Part model, mm, in its own coordinate system. A direction names the side the tool comes from. Round coordinates to 2 decimals unless told otherwise and drop trailing zeros. Order: outer loops, then holes, each group sorted by start corner. A loop starts at its lowest first (then second) coordinate and runs counter-clockwise, first axis right, second up. Notation, with made-up numbers: (-30.5, -12) -> (-17.5, -12) arc R9 ccw to (-17.5, 3) -> close; hole circle Ø9 at (-10.5, 71). An arc over 180 degrees is marked (long way). Answer as a JSON object with one key per item and string values. Group by question number.
```python
from build123d import *

# Parameters (mm, degrees)
SKETCH1_W           = 90
SKETCH1_H           = 140
BOSS_EXTRUDE1_DEPTH = 5
SKETCH2_W           = 80
SKETCH2_H           = 85
CUT_EXTRUDE1_DEPTH  = 2
SKETCH3_W           = 90
SKETCH3_H           = 3
BOSS_EXTRUDE2_DEPTH = 50
SKETCH4_W           = 2
SKETCH4_H           = 134
BOSS_EXTRUDE3_DEPTH = 50
SKETCH5_R           = 4
CUT_EXTRUDE2_DEPTH  = 3
SKETCH6_R           = 4
CUT_EXTRUDE3_DEPTH  = 3


with BuildPart() as part:
    # Sketch1 → Boss-Extrude1 (new body)
    with BuildSketch(Plane(origin=(0, 0, 0), x_dir=(1, 0, 0), z_dir=(0, 1, 0))):
        Rectangle(SKETCH1_W, SKETCH1_H)
    extrude(amount=BOSS_EXTRUDE1_DEPTH)

    # Sketch2 → Cut-Extrude1 (cut)
    with BuildSketch(Plane(origin=(0, 5, 0), x_dir=(1, 0, 0), z_dir=(0, 1, 0))):
        Rectangle(SKETCH2_W, SKETCH2_H)
    extrude(amount=-CUT_EXTRUDE1_DEPTH, mode=Mode.SUBTRACT)

    # Sketch3 → Boss-Extrude2 (add)
    with BuildSketch(Plane(origin=(0, 5, 0), x_dir=(1, 0, 0), z_dir=(0, 1, 0))):
        with Locations((0, -68.5)):
            Rectangle(SKETCH3_W, SKETCH3_H)
        with Locations((0, 68.5)):
            Rectangle(SKETCH3_W, SKETCH3_H)
    extrude(amount=BOSS_EXTRUDE2_DEPTH)

    # Sketch4 → Boss-Extrude3 (add)
    with BuildSketch(Plane(origin=(0, 5, 0), x_dir=(1, 0, 0), z_dir=(0, 1, 0))):
        with Locations((-44, 0)):
            Rectangle(SKETCH4_W, SKETCH4_H)
        with Locations((44, 0)):
            Rectangle(SKETCH4_W, SKETCH4_H)
    extrude(amount=BOSS_EXTRUDE3_DEPTH)

    # Sketch5 → Cut-Extrude2 (cut)
    with BuildSketch(Plane.XY.offset(70)):
        with Locations((0, 25)):
            Circle(SKETCH5_R)
        with Locations((28, 25)):
            Circle(SKETCH5_R)
        with Locations((-28, 25)):
            Circle(SKETCH5_R)
    extrude(amount=-CUT_EXTRUDE2_DEPTH, mode=Mode.SUBTRACT)

    # Sketch6 → Cut-Extrude3 (cut)
    with BuildSketch(Plane(origin=(0, 0, -70), x_dir=(-1, 0, 0), z_dir=(0, 0, -1))):
        with Locations((-25, 25)):
            Circle(SKETCH6_R)
        with Locations((25, 25)):
            Circle(SKETCH6_R)
    extrude(amount=-CUT_EXTRUDE3_DEPTH, mode=Mode.SUBTRACT)


solid = part.part
```
Q1. Band-saw the part on D-D (z = 58). List the corners of the cut face in (x, y), plus the area to 3 significant figures.
Q2. Two-plate mould, pull along Y, no slides. Class faces 1 (the flat face through (-1, 3, -1)), 2 (the cylindrical face through (25.521, 28.966, -68.521)), 3 (the flat face through (-1, 30, 67)): +Y half, -Y half, draft (parallel to the pull), parting line (faces both ways), or undercut.
Q3. Drop flat-ended pins along their axis: pin 1 Ø3 at (x, z) = (28.5, -15.5) entering from +Y; pin 2 Ø10.5 at (x, y) = (28, 25) entering from -Z; pin 3 Ø5 at (x, z) = (0, -50) entering from +Y; pin 4 Ø7 at (x, y) = (-28, 25) entering from +Z. Give the stop position or say it passes through.
Q4. Wall check: line 1 (Z direction, x = -30, y = 15); line 2 (X direction, y = 23.5, z = -10.5); line 3 (Y direction, x = -28, z = 67.8). Give the ranges that are in metal, low to high. Write a range as [from, to].
Q5. Band-saw the part on B-B (x = -14). List the corners of the cut face in (y, z), plus the area to 3 significant figures.
Q6. Band-saw the part on A-A (x = 0). List the corners of the cut face in (y, z).
Q7. Which spindle directions (+Z, -Z, +X, -X, +Y, -Y) get a long thin tool onto all of the face, cutting with end or side? Do faces 4 (the flat face through (45, 27, 1)), 5 (the cylindrical face through (-28.521, 28.966, 68.521)), 6 (the flat face through (-1, 30, -67)), 7 (the flat face through (-1, 33, 70)), 8 (the cylindrical face through (-24.479, 28.966, -68.521)). Say none if no direction does.
Q8. Band-saw the part on C-C (y = 39). List the corners of the cut face in (x, z), plus the area to 3 significant figures.
Completed:
{
 "1": {"outline": "(-45, 0) -> (45, 0) -> (45, 55) -> (43, 55) -> (43, 5) -> (-43, 5) -> (-43, 55) -> (-45, 55) -> close", "area": "650 mm2"},
 "2": {"face 1": "+Y half", "face 2": "undercut", "face 3": "draft"},
 "3": {"pin 1": "y = 3", "pin 2": "z = -70", "pin 3": "y = 5", "pin 4": "z = -67"},
 "4": {"line 1": "[-70, -67], [67, 70]", "line 2": "[-45, -43], [43, 45]", "line 3": "[0, 21], [29, 55]"},
 "5": {"outline": "(0, -70) -> (55, -70) -> (55, -67) -> (5, -67) -> (5, -42.5) -> (3, -42.5) -> (3, 42.5) -> (5, 42.5) -> (5, 67) -> (55, 67) -> (55, 70) -> (0, 70) -> close", "area": "830 mm2"},
 "6": {"outline": "(0, -70) -> (55, -70) -> (55, -67) -> (5, -67) -> (5, -42.5) -> (3, -42.5) -> (3, 42.5) -> (5, 42.5) -> (5, 67) -> (21, 67) -> (21, 70) -> (0, 70) -> close; (29, 67) -> (55, 67) -> (55, 70) -> (29, 70) -> close"},
 "7": {"face 4": "+Z, -Z, +X, +Y, -Y", "face 5": "+Z", "face 6": "+Y", "face 7": "+Z, +X, -X, +Y, -Y", "face 8": "-Z"},
 "8": {"outline": "(-45, -70) -> (45, -70) -> (45, 70) -> (-45, 70) -> close; hole (-43, -67) -> (43, -67) -> (43, 67) -> (-43, 67) -> close", "area": "1,080 mm2"}
}
